Could you check a few things on this model? Use its own coordinates, in mm. A direction names the side the tool comes from. Coordinates: 2 decimals unless noted, no trailing zeros. Loops run counter-clockwise (first coordinate to the right, second up) from the corner with the lowest first, then second, coordinate; pieces in that order, holes last. Notation, with made-up numbers: (47.5, 21.25) - (54.5, 21.25) arc R24 ccw to (54.5, 31.25) - close; hole circle Ø1 at (87.25, 0). An arc over 180 degrees is marked (long way). One line per item, written item: value. Start each with the question number.
(1) If we section it at C-C on z = 3.5: Write out the boundary of the cut face in (x, y), then the cut area to 3 significant figures.
(2) If I drill on line 1 along Z through (x, y) = (-12.25, 186.5); line 2 along X through (y, z) = (205, -4); line 3 along X through (y, z) = (198, -3.25), over which ranges is the centre line in solid material (lowest first)? Write a range as from..to.
(3) If we section it at A-A on y = 163: Count the separate pieces of the cut face and the enclosed holes in it, then the cut area to 3 significant figures.
(4) If we mould it in two halves opening along X, with no side actions, what happens to faces 1 (the face through (-7.41, 185.1, 5.46)), 2 (the face through (0.447, 184.056, -0.138)), 3 (the face through (-17.455, 182.201, 0.138))? For each: pulls with the +X half, pulls with the -X half, needs draft (parallel to the pull), parting line crosses it, or undercut.
(5) If we section it at B-B on z = -6.25: Write out the boundary of the cut face in (x, y), then the cut area to 3 significant figures.
(6) I'm going to push flat-ended pins straight in: P1, Ø6, axis at y = 198, z = -3.5, coming from the +X side; P2, Ø1, axis at y = 172, z = 4.5, coming from the +X side; P3, Ø6, axis at x = -14, z = 2.5, coming from the -Y side. Where does each tip first touch, or does it pass through?
(7) On a 3-axis mill with a long thin cutter (end or side, diameter ignored), from which of +Z, -Z, +X, -X, +Y, -Y can I reach the whole of each face in a straight line? I mean faces 4 (the face through (-3.75, 148.94, 0.66)), 5 (the face through (-3.449, 183.613, -3.613)), 6 (the face through (-6.14, 148.69, 0.66)). Say none if no direction works.
```python
from build123d import *

# Parameters (mm, degrees)
SKETCH3_R               = 9
BOSS_EXTRUDE1_DEPTH     = 69
CUT_EXTRUDE1_DEPTH      = 220.929043992
CUT_EXTRUDE1_DEPTH_BACK = 220.929043992
CUT_EXTRUDE2_DEPTH      = 219.597133119
CUT_EXTRUDE2_DEPTH_BACK = 219.597133119
BOSS_EXTRUDE3_DEPTH     = 1.2
SKETCH8_R               = 1.6
SKETCH8_R_2             = 1.4
CUT_EXTRUDE3_DEPTH      = 74.512311312
CUT_EXTRUDE3_DEPTH_BACK = 74.512311312
CUT_EXTRUDE4_DEPTH      = 73.514420315


with BuildPart() as part:
    # Sketch3 → Boss-Extrude1 (new body)
    with BuildSketch(Plane(origin=(-12.082314344, 217.636022384, 0), x_dir=(-0.9946657577296572, -0.10315052302381673, 0), z_dir=(0.10315052302381673, -0.9946657577296572, 0))):
        with Locations(Location((0, 0, 0), (0, 0, 180))):
            Circle(SKETCH3_R)
    extrude(amount=BOSS_EXTRUDE1_DEPTH)

    # Sketch4 → Cut-Extrude1 (cut, two sides)
    with BuildSketch(Plane(origin=(10.375761543, 1.076004901, 0), x_dir=(0.10315052302381672, -0.9946657577296572, 0), z_dir=(-0.9946657577296572, -0.10315052302381673, 0))) as cut_extrude1_sk:
        with BuildLine():
            Line((-217.721396158, 9), (-212.721396158, 9))
            ThreePointArc((-212.721396158, 9), (-216.387282909, 0), (-212.721396158, -9))
            Line((-212.721396158, -9), (-217.721396158, -9))
            Line((-217.721396158, -9), (-217.721396158, 9))
        make_face()
    extrude(amount=CUT_EXTRUDE1_DEPTH, mode=Mode.SUBTRACT)
    extrude(cut_extrude1_sk.sketch, amount=-CUT_EXTRUDE1_DEPTH_BACK, mode=Mode.SUBTRACT)

    # Sketch5 → Cut-Extrude2 (cut, two sides)
    with BuildSketch(Plane(origin=(10.375761543, 1.076004901, 0), x_dir=(0.10315052302381672, -0.9946657577296572, 0), z_dir=(-0.9946657577296572, -0.10315052302381673, 0))) as cut_extrude2_sk:
        Polygon((-148.721396158, 0), (-157.721396158, 9), (-148.721396158, 9), align=None)
    extrude(amount=CUT_EXTRUDE2_DEPTH, mode=Mode.SUBTRACT)
    extrude(cut_extrude2_sk.sketch, amount=-CUT_EXTRUDE2_DEPTH_BACK, mode=Mode.SUBTRACT)

    # Sketch7 → Boss-Extrude3 (add, symmetric)
    with BuildSketch(Plane(origin=(10.375761543, 1.076004901, 0), x_dir=(0.10315052302381672, -0.9946657577296572, 0), z_dir=(-0.9946657577296572, -0.10315052302381673, 0))):
        with BuildLine():
            Line((-151.519146847, 0.112209978), (-148.721396158, 0))
            Line((-148.721396158, 0), (-148.721396158, -2.8))
            Line((-148.721396158, -2.8), (-146.296525027, 1.4))
            ThreePointArc((-146.296525027, 1.4), (-149.391739784, 2.718573049), (-151.519146847, 0.112209978))
        make_face()
    extrude(amount=BOSS_EXTRUDE3_DEPTH, both=True)

    # Sketch8 → Cut-Extrude3 (cut, two sides)
    with BuildSketch(Plane(origin=(-12.082314344, 217.636022384, 0), x_dir=(-0.9946657577296572, -0.10315052302381673, 0), z_dir=(0.10315052302381673, -0.9946657577296572, 0))) as cut_extrude3_sk:
        with Locations(Location((-3.6, 3, 0), (0, 0, 180))):
            Circle(SKETCH8_R)
        with Locations(Location((3.6, 3, 0), (0, 0, 180))):
            Circle(SKETCH8_R)
        with Locations(Location((0, -6, 0), (0, 0, 180))):
            Circle(SKETCH8_R_2)
    extrude(amount=CUT_EXTRUDE3_DEPTH, mode=Mode.SUBTRACT)
    extrude(cut_extrude3_sk.sketch, amount=-CUT_EXTRUDE3_DEPTH_BACK, mode=Mode.SUBTRACT)

    # Sketch9 → Cut-Extrude4 (cut, through all)
    with BuildSketch(Plane(origin=(-15.340689799, 147.9280802, 0), x_dir=(0.9946657577296572, 0.10315052302381673, 0), z_dir=(0.10315052302381673, -0.9946657577296572, 0))):
        with BuildLine():
            Line((6.30829956, -8), (14.554510811, -8))
            ThreePointArc((14.554510811, -8), (10.431405186, -9), (6.30829956, -8))
        make_face()
        with BuildLine():
            Line((6.30829956, 8), (14.554510811, 8))
            ThreePointArc((14.554510811, 8), (10.431405186, 9), (6.30829956, 8))
        make_face()
    extrude(amount=-CUT_EXTRUDE4_DEPTH, mode=Mode.SUBTRACT)


solid = part.part
```
Values:
1. outline: (-20.14, 214.97) - (-13.57, 151.63) - (2.92, 153.34) - (-3.65, 216.68) - close
1. area: 1,060 mm2
2. line 1: z = -8..-4.58, -1.42..8
2. line 2: x = -18.88..-15.65, -13.14..-8.41, -5.9..-2.67
2. line 3: x = -18.48..-15.25, -12.08..-8.02, -4.84..-1.61
3. separate pieces: 1
3. enclosed holes: 3
3. area: 222 mm2
4. face 1: undercut
4. face 2: pulls with the +X half
4. face 3: pulls with the -X half
5. outline: (-18.22, 214.03) - (-11.41, 148.34) - (1.48, 149.67) - (-5.34, 215.37) - close
5. area: 855 mm2
6. P1: stops at x = -0.88
6. P2: stops at x = 0.76
6. P3: stops at y = 148.08
7. face 4: +Z, +X
7. face 5: none
7. face 6: +Z, -Y
